Read the model definition and answer for the solid it produces. Units are mm, in the model's axes. Coordinates: 2 decimals unless noted, no trailing zeros. Loops run counter-clockwise (first coordinate to the right, second up) from the corner with the lowest first, then second, coordinate; pieces in that order, holes last. Notation, with made-up numbers: (37.25, 36.5) -> (87.25, 36.5) arc R27 cw to (87.25, 56.5) -> close; hole circle Ø5 at (-27.5, 87). An arc over 180 degrees is marked (long way). Answer as CSV lines item,"result".
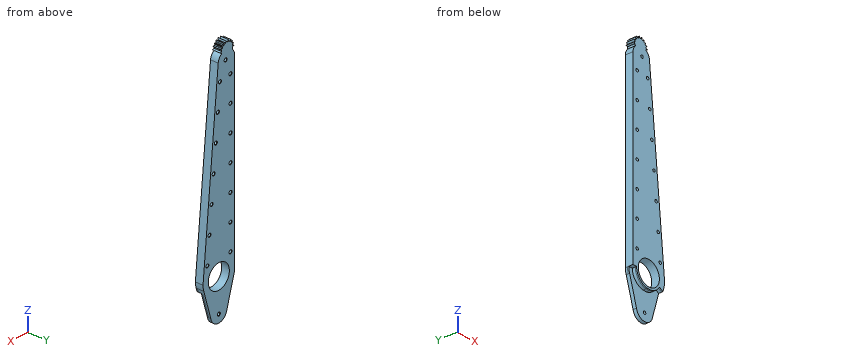
```python
from build123d import *
from build123d.topology import SkipClean

# Parameters (mm, degrees)
EXTRUDE_1_DEPTH               = 15
CUT_EXTRUDE_1_DEPTH           = 4
SKETCH_3_R                    = 14
CUT_EXTRUDE_2_DEPTH           = 227.475164201
EXTRUDE_4_DEPTH               = 15
SKETCH_11_W                   = 17
SKETCH_11_H                   = 10
SKETCH_14_W                   = 6
SKETCH_14_H                   = 10
CUT_REVOLVE_4_ANGLE           = 60
CUT_REVOLVE_4_OTHER_WAY_ANGLE = 90
SKETCH_16_W                   = 9.609453317
SKETCH_16_H                   = 10
CUT_EXTRUDE_4_DEPTH           = 5
SKETCH_17_W                   = 9.609453317
SKETCH_17_H                   = 10
CUT_EXTRUDE_5_DEPTH           = 5
CUT_EXTRUDE_6_DEPTH           = 7.5
EXTRUDE_START                 = 1.5
EXTRUDE_6_DEPTH               = 1.5
SKETCH_21_R                   = 5
SKETCH_21_R_2                 = 14
EXTRUDE_7_DEPTH               = 1.5
HOLE_WIZARD_M4_1_D            = 3.3
HOLE_WIZARD_M4_1_DEPTH        = 9
HOLE_WIZARD_M4_1_CSINK_D      = 4.05
HOLE_WIZARD_M4_1_CSINK_ANGLE  = 90
SKETCH_25_R                   = 5
CUT_EXTRUDE_7_DEPTH           = 5
EXTRUDE_8_DEPTH               = 9


with BuildPart() as part:
    # 草图1 → 凸台-拉伸1 (new body)
    with BuildSketch(Plane(origin=(0, 0, 0), x_dir=(1, 0, 0), z_dir=(0, 1, 0))):
        with BuildLine():
            Line((-21, 0), (-21, -215))
            ThreePointArc((-21, -215), (-18.071067812, -222.071067812), (-11, -225))
            Line((-11, -225), (-9.110127779, -225))
            ThreePointArc((-9.110127779, -225), (-2.375625019, -222.392325249), (0.846599179, -215.929294516))
            Line((0.846599179, -215.929294516), (21, 0))
            ThreePointArc((21, 0), (0, 21), (-21, 0))
        make_face()
    extrude(amount=EXTRUDE_1_DEPTH)

    # 草图2 → 切除-拉伸1 (cut)
    with BuildSketch(Plane.XZ):
        with BuildLine():
            Line((-6.487547308, 24.545681698), (-15.16946684, 197.954199749))
            ThreePointArc((-15.16946684, 197.954199749), (-9.006726896, 204.766554422), (-2.194372223, 198.603814478))
            Line((-2.194372223, 198.603814478), (6.487547308, 25.195296427))
            ThreePointArc((6.487547308, 25.195296427), (0.324807364, 18.382941754), (-6.487547308, 24.545681698))
        make_face()
    extrude(amount=-CUT_EXTRUDE_1_DEPTH, mode=Mode.SUBTRACT)

    # 草图3 → 切除-拉伸2 (cut, through all)
    with BuildSketch(Plane(origin=(0, 0, 0), x_dir=(-1, 0, 0), z_dir=(0, -1, 0))):
        with Locations(Location((0, 0, 0), (0, 0, 90))):
            Circle(SKETCH_3_R)
    extrude(amount=-CUT_EXTRUDE_2_DEPTH, mode=Mode.SUBTRACT)

    # 草图7 → 凸台-拉伸4 (add)
    with BuildSketch(Plane(origin=(0, 0, 0), x_dir=(1, 0, 0), z_dir=(0, 1, 0))):
        with BuildLine():
            Line((-10.693069191, 38.039100971), (-19.9158097, 6.66036966))
            ThreePointArc((-19.9158097, 6.66036966), (0, 21), (19.9158097, 6.66036966))
            Line((19.9158097, 6.66036966), (10.693069191, 38.039100971))
            ThreePointArc((10.693069191, 38.039100971), (0, 47.113526612), (-10.693069191, 38.039100971))
        make_face()
    extrude(amount=EXTRUDE_4_DEPTH)

    # 草图11 → 切除-旋转3 (revolve, cut)
    with BuildSketch(Plane(origin=(0, 0, 0), x_dir=(0, 0, -1), z_dir=(1, 0, 0)), mode=Mode.PRIVATE) as cut_revolve_3_sk:
        with Locations((51.539100971, 7.5)):
            Rectangle(SKETCH_11_W, SKETCH_11_H)
    revolve(cut_revolve_3_sk.sketch.rotate(Axis((0, 15, -38.039100971), (0, -1, 0)), 180), axis=Axis((0, 15, -38.039100971), (0, -1, 0)), mode=Mode.SUBTRACT)

    # 草图14 → 切除-旋转4 (revolve, cut)
    with BuildSketch(Plane(origin=(0, 0, 0), x_dir=(0, 0, -1), z_dir=(1, 0, 0))):
        with Locations((19.26034239, 7.5)):
            Rectangle(SKETCH_14_W, SKETCH_14_H)
    revolve(axis=Axis((0, 15, 0), (0, -1, 0)), revolution_arc=CUT_REVOLVE_4_ANGLE, mode=Mode.SUBTRACT)

    # 草图14 → 切除-旋转4 other way (revolve, cut)
    with BuildSketch(Plane(origin=(0, 0, 0), x_dir=(0, 0, -1), z_dir=(1, 0, 0))):
        with Locations((19.26034239, 7.5)):
            Rectangle(SKETCH_14_W, SKETCH_14_H)
    revolve(axis=Axis((0, 15, 0), (0, 1, 0)), revolution_arc=CUT_REVOLVE_4_OTHER_WAY_ANGLE, mode=Mode.SUBTRACT)

    # 草图16 → 切除-拉伸4 (cut)
    with BuildSketch(Plane(origin=(20.13407913, 0, -5.917746812), x_dir=(-0.2819890835944097, 0, -0.9594176133121516), z_dir=(0.9594176133121516, 0, -0.2819890835944097))):
        with Locations((12.229144047, 7.5)):
            Rectangle(SKETCH_16_W, SKETCH_16_H)
    extrude(amount=-CUT_EXTRUDE_4_DEPTH, mode=Mode.SUBTRACT)

    # 草图17 → 切除-拉伸5 (cut)
    with BuildSketch(Plane(origin=(-20.13407913, 0, -5.917746812), x_dir=(-0.28198908359441, 0, 0.9594176133121515), z_dir=(-0.9594176133121515, 0, -0.28198908359441))):
        with Locations((-12.229144047, 7.5)):
            Rectangle(SKETCH_17_W, SKETCH_17_H)
    extrude(amount=-CUT_EXTRUDE_5_DEPTH, mode=Mode.SUBTRACT)

    # 草图20 → 切除-拉伸6 (cut)
    with BuildSketch(Plane.XZ):
        with BuildLine():
            Line((21, 0), (0.846599179, 215.929294516))
            ThreePointArc((0.846599179, 215.929294516), (-2.375625019, 222.392325249), (-9.110127779, 225))
            Line((-9.110127779, 225), (-11, 225))
            ThreePointArc((-11, 225), (-18.071067812, 222.071067812), (-21, 215))
            Line((-21, 215), (-21, 0))
            ThreePointArc((-21, 0), (-20.727180268, -3.374018102), (-19.9158097, -6.66036966))
            Line((-19.9158097, -6.66036966), (-10.693069191, -38.039100971))
            ThreePointArc((-10.693069191, -38.039100971), (0, -47.113526612), (10.693069191, -38.039100971))
            Line((10.693069191, -38.039100971), (19.9158097, -6.66036966))
            ThreePointArc((19.9158097, -6.66036966), (20.727180268, -3.374018102), (21, 0))
        make_face()
    extrude(amount=-CUT_EXTRUDE_6_DEPTH, mode=Mode.SUBTRACT)

    # 草图22 → 凸台-拉伸6 (add)
    with BuildSketch(Plane.XZ.offset(-12.5).offset(EXTRUDE_START)):
        with BuildLine():
            Line((-19.9158097, -6.66036966), (-10.693069191, -38.039100971))
            ThreePointArc((-10.693069191, -38.039100971), (0, -47.113526612), (10.693069191, -38.039100971))
            Line((10.693069191, -38.039100971), (18.700124508, -10.796521919))
            Line((18.700124508, -10.796521919), (14.081869584, -8.130171195))
            ThreePointArc((14.081869584, -8.130171195), (8.995321483, -13.545586959), (2.030780118, -16.133030303))
            ThreePointArc((2.030780118, -16.133030303), (0, -16.039100971), (-2.030780118, -16.133030303))
            ThreePointArc((-2.030780118, -16.133030303), (-12.194669218, -10.755871759), (-16.26034239, 0))
            Line((-16.26034239, 0), (-21, 0))
            ThreePointArc((-21, 0), (-20.727180268, -3.374018102), (-19.9158097, -6.66036966))
        make_face()
    extrude(amount=-EXTRUDE_6_DEPTH)

    # 草图21 → 凸台-拉伸7 (add)
    # profile 1 of 2: a face of its own
    with SkipClean():  # the faces are left unmerged after this step: merging them gives an invalid solid
        with BuildSketch(Plane.XZ.offset(-7.5).offset(EXTRUDE_START)):
            with Locations(Location((0, -38.039100971, 0), (0, 0, 270))):
                Circle(SKETCH_21_R)
        # profile 2 of 2: a face of its own
        with BuildSketch(Plane.XZ.offset(-7.5).offset(EXTRUDE_START)):
            with BuildLine():
                Line((-21, 0), (-16.26034239, 0))
                ThreePointArc((-16.26034239, 0), (-12.194669218, -10.755871759), (-2.030780118, -16.133030303))
                ThreePointArc((-2.030780118, -16.133030303), (0, -16.039100971), (2.030780118, -16.133030303))
                ThreePointArc((2.030780118, -16.133030303), (8.995321483, -13.545586959), (14.081869584, -8.130171195))
                Line((14.081869584, -8.130171195), (18.700124508, -10.796521919))
                Line((18.700124508, -10.796521919), (19.9158097, -6.66036966))
                ThreePointArc((19.9158097, -6.66036966), (20.727180268, -3.374018102), (21, 0))
                Line((21, 0), (0.846599179, 215.929294516))
                ThreePointArc((0.846599179, 215.929294516), (-2.375625019, 222.392325249), (-9.110127779, 225))
                Line((-9.110127779, 225), (-11, 225))
                ThreePointArc((-11, 225), (-18.071067812, 222.071067812), (-21, 215))
                Line((-21, 215), (-21, 0))
            make_face()
            with Locations(Location((0, 0, 0), (0, 0, 270))):
                Circle(SKETCH_21_R_2, mode=Mode.SUBTRACT)
        extrude(amount=-EXTRUDE_7_DEPTH)

    # M4 螺纹孔1
    with Locations(Plane(origin=(0, 15, 0), x_dir=(1, 0, 0), z_dir=(0, 1, 0))):
        with Locations((-1.550565844, -196.226581502), (-4.338449392, -226.096762374), (-9.110127779, -215), (15.176735444, -17.005496271), (0, 38.039100971), (-15.5, -18.398087501), (-15.5, -48.398087501), (-15.5, -78.398087501), (-15.5, -108.398087501), (-15.5, -138.398087501), (-15.5, -168.398087501), (-15.5, -198.398087501), (12.388851896, -46.875677143), (9.600968348, -76.745858014), (6.8130848, -106.616038886), (4.025201252, -136.486219758), (1.237317704, -166.35640063)):
            CounterSinkHole(HOLE_WIZARD_M4_1_D / 2, HOLE_WIZARD_M4_1_CSINK_D / 2, depth=HOLE_WIZARD_M4_1_DEPTH, counter_sink_angle=HOLE_WIZARD_M4_1_CSINK_ANGLE)

    # 草图25 → 切除-拉伸7 (cut)
    with BuildSketch(Plane.XZ.offset(-6)):
        with Locations((0, -38.039100971)):
            Circle(SKETCH_25_R)
    extrude(amount=-CUT_EXTRUDE_7_DEPTH, mode=Mode.SUBTRACT)

    # 草图26 → 凸台-拉伸8 (add)
    with BuildSketch(Plane(origin=(0, 15, 0), x_dir=(1, 0, 0), z_dir=(0, 1, 0))):
        with BuildLine():
            Line((-18.307809651, -224.266369979), (-20.284097218, -225))
            Line((-20.284097218, -225), (-18.307809651, -225.733630021))
            ThreePointArc((-18.307809651, -225.733630021), (-18.232961751, -226.275366307), (-18.118011048, -226.810031388))
            Line((-18.118011048, -226.810031388), (-19.724197646, -228.175348261))
            Line((-19.724197646, -228.175348261), (-17.616178559, -228.188804821))
            ThreePointArc((-17.616178559, -228.188804821), (-17.360559817, -228.672270922), (-17.069675262, -229.135376297))
            Line((-17.069675262, -229.135376297), (-18.112031083, -230.967702659))
            Line((-18.112031083, -230.967702659), (-16.126538687, -230.259362699))
            ThreePointArc((-16.126538687, -230.259362699), (-15.720980497, -230.626245467), (-15.289247061, -230.961933794))
            Line((-15.289247061, -230.961933794), (-15.642048609, -233.040264042))
            Line((-15.642048609, -233.040264042), (-14.018562591, -231.695563814))
            ThreePointArc((-14.018562591, -231.695563814), (-13.511981254, -231.901611775), (-12.991472361, -232.069394086))
            Line((-12.991472361, -232.069394086), (-12.612166563, -234.14305092))
            Line((-12.612166563, -234.14305092), (-11.546503297, -232.324181118))
            ThreePointArc((-11.546503297, -232.324181118), (-11, -232.344541845), (-10.453496703, -232.324181118))
            Line((-10.453496703, -232.324181118), (-9.387833437, -234.14305092))
            Line((-9.387833437, -234.14305092), (-9.008527639, -232.069394086))
            ThreePointArc((-9.008527639, -232.069394086), (-8.488018746, -231.901611775), (-7.981437409, -231.695563814))
            Line((-7.981437409, -231.695563814), (-6.357951391, -233.040264042))
            Line((-6.357951391, -233.040264042), (-6.710752939, -230.961933794))
            ThreePointArc((-6.710752939, -230.961933794), (-6.279019503, -230.626245467), (-5.873461313, -230.259362699))
            Line((-5.873461313, -230.259362699), (-3.887968917, -230.967702659))
            Line((-3.887968917, -230.967702659), (-4.930324738, -229.135376297))
            ThreePointArc((-4.930324738, -229.135376297), (-4.639440183, -228.672270922), (-4.383821441, -228.188804821))
            Line((-4.383821441, -228.188804821), (-2.275802354, -228.175348261))
            Line((-2.275802354, -228.175348261), (-3.881988952, -226.810031388))
            ThreePointArc((-3.881988952, -226.810031388), (-3.767038249, -226.275366307), (-3.692190349, -225.733630021))
            Line((-3.692190349, -225.733630021), (-1.715902782, -225))
            Line((-1.715902782, -225), (-3.692190349, -224.266369979))
            ThreePointArc((-3.692190349, -224.266369979), (-11, -217.655458155), (-18.307809651, -224.266369979))
        make_face()
    extrude(amount=-EXTRUDE_8_DEPTH)


solid = part.part
```
Q1. A cutting plane is placed at B-B, the plane z = 41. Write down the section's boundary in (x, y).
Results:
outline,"(-21, 6) -> (17.17, 6) -> (17.17, 15) -> (-21, 15) -> close"
Q2. A cutting plane is placed at A-A, the plane z = 72. Write down the section's boundary in (x, y).
Results:
outline,"(-21, 6) -> (14.28, 6) -> (14.28, 15) -> (-21, 15) -> close"
Q3. Find the intervals of material crossed by probe 1 along Z at (x, y) = (-10, 7.25); probe 2 along Z at (x, y) = (-1.5, 8); probe 3 along X at (y, z) = (7, 17), in increasing order. Write a range as [from, to].
Results:
probe 1,"z = [-12.82, -9.8], [9.8, 213.61], [216.39, 233.1]"
probe 2,"z = [-16.09, -13.92], [13.92, 194.58], [197.88, 221.49]"
probe 3,"x = [-21, -16.38], [-14.62, 13.53], [16.83, 19.41]"
Q4. Given pin 1 Ø2 at (x, y) = (-9.5, 10.5) entering from -Z; pin 2 Ø2 at (x, y) = (-8.5, 8) entering from -Z, each flat-ended and moving along its own axis, determine where each tip first touches the part or whether it passes through.
Results:
pin 1,"stops at z = -42.83"
pin 2,"stops at z = -14.43"
